The model under review builds one solid part; all positions refer to its coordinate system, in mm. A direction names the side the tool comes from. Give positions to 0.01 mm unless a question says otherwise; leave off trailing zeros. Write each loop counter-clockwise with the first axis right and the second up, starting at its lowest first coordinate (ties: lowest second). Pieces come first, ordered by that corner, then holes.
from build123d import *

# Parameters (mm, degrees)
F_4_0_4_DIAMETER_HOLE1_D = 4


with BuildPart() as part:
    # Sketch1 → Revolve1 (revolve)
    with BuildSketch(Plane(origin=(0, 0, 0), x_dir=(0, 0, -1), z_dir=(1, 0, 0)), mode=Mode.PRIVATE) as revolve1_sk:
        Polygon((0, 0), (0, 6.5), (-1, 6.5), (-3, 4.5), (-5, 6.5), (-6, 6.5), (-6, 0), align=None)
    revolve(revolve1_sk.sketch.rotate(Axis((0, 0, 55), (0, 0, -1)), 90), axis=Axis((0, 0, 55), (0, 0, -1)))

    # Ø4.0 (4) Diameter Hole1 (through all)
    with Locations(Plane.XY.offset(6)):
        with Locations((0, 0)):
            Hole(F_4_0_4_DIAMETER_HOLE1_D / 2)


solid = part.part
1) Consider section C-C, the plane z = 1.75. Give the boundary of the cut face in (x, y), then the cut area to 3 significant figures.
2) Consider section D-D, the plane z = 2.5. Give the boundary of the cut face in (x, y).
3) Consider section A-A, the plane y = 0. Give the boundary of the cut face in (x, z).
4) The part is to be moulded in two halves that separate along X. For faces 1 (the cylindrical face through (-5.158, 3.955, 0.507)), 2 (the cylindrical face through (0, -2, 3)), 3 (the flat face through (1, -2, 6)), say which applies: +X half, -X half, draft (parallel to the pull), parting line (faces both ways), or undercut.
5) To check wall thickness, follow probe 1 along Y at (x, z) = (0, 0.9); probe 2 along X at (y, z) = (-0.75, 3.45); probe 3 along X at (y, z) = (0.5, 2.45). State the ranges of each line that lie inside material, in increasing order.
6) Tool access review of faces 4 (the conical face through (2.134, 4.103, 3.125)), 5 (the flat face through (-1, -2, 0)): name each direction out of +Z, -Z, +X, -X, +Y, -Y from which nothing blocks a thin tool from reaching the whole face with its end or side.
Answer block:
1. outline: circle Ø11.5 at (0, 0); hole circle Ø4 at (0, 0)
1. area: 91.3 mm2
2. outline: circle Ø10 at (0, 0); hole circle Ø4 at (0, 0)
3. outline: (-6.5, 0) - (-2, 0) - (-2, 6) - (-6.5, 6) - (-6.5, 5) - (-4.5, 3) - (-6.5, 1) - close; (2, 0) - (6.5, 0) - (6.5, 1) - (4.5, 3) - (6.5, 5) - (6.5, 6) - (2, 6) - close
4. face 1: parting line
4. face 2: undercut
4. face 3: draft
5. probe 1: y = -6.5 to -2, 2 to 6.5
5. probe 2: x = -4.89 to -1.85, 1.85 to 4.89
5. probe 3: x = -5.03 to -1.94, 1.94 to 5.03
6. face 4: none
6. face 5: -Z, +X, -X, +Y, -Y
